```python
from build123d import *

# Parameters (mm, degrees)
SKETCH1_W           = 1500
SKETCH1_H           = 400
BOSS_EXTRUDE1_DEPTH = 6
BOSS_EXTRUDE2_DEPTH = 500
SKETCH3_W           = 10
SKETCH3_H           = 500
CUT_EXTRUDE1_DEPTH  = 4


with BuildPart() as part:
    # Sketch1 → Boss-Extrude1 (new, symmetric)
    with BuildSketch(Plane(origin=(0, 0, 0), x_dir=(1, 0, 0), z_dir=(0, 1, 0))):
        Rectangle(SKETCH1_W, SKETCH1_H)
    extrude(amount=BOSS_EXTRUDE1_DEPTH, both=True)

    # Sketch2 → Boss-Extrude2 (add)
    with BuildSketch(Plane(origin=(0, 6, 0), x_dir=(1, 0, 0), z_dir=(0, 1, 0))):
        Polygon((738, 188), (750, 188), (750, 200), (-750, 200), (-750, -200), (750, -200), (750, -188), (738, -188), (-738, -188), (-738, 188), align=None)
    extrude(amount=BOSS_EXTRUDE2_DEPTH)

    # Sketch3 → Cut-Extrude1 (cut)
    with BuildSketch(Plane.XY.offset(-188)):
        with Locations((440.2, 256)):
            Rectangle(SKETCH3_W, SKETCH3_H)
    cut_extrude1 = extrude(amount=-CUT_EXTRUDE1_DEPTH, mode=Mode.SUBTRACT)

    # Mirror1: Cut-Extrude1 across plane
    add(cut_extrude1.mirror(Plane.XY), mode=Mode.SUBTRACT)


solid = part.part
```
Part model, mm, in its own coordinate system. A direction names the side the tool comes from. Coordinates: 2 decimals unless noted, no trailing zeros. Write each loop counter-clockwise with the first axis right and the second up, starting at its lowest first coordinate (ties: lowest second). Pieces come first, ordered by that corner, then holes.
Item 1: Slice it at B-B (z = -5). Write the cut outline in (x, y), and give its area (3 significant figures).
Item 2: Mould opens along Z. For faces 1 (the face through (-143, 252, 188)), 2 (the face through (-10, 254, 200)), 3 (the face through (-4, 506, -194)), 4 (the face through (10, 246, -200)) say: released by +Z, released by -Z, zero draft, split by the parting line, or undercut.
Item 3: Which spindle directions (+Z, -Z, +X, -X, +Y, -Y) get a long thin tool onto all of the face, cutting with end or side? Do faces 5 (the face through (-10, -6, -3)), 6 (the face through (-738, 252, 3)). Say none if no direction does.
Item 4: Slice it at A-A (x = 526). Write the cut outline in (y, z), and give its area (3 significant figures).
Item 5: Probe line 1 (Z direction, x = -198, y = 236.5); line 2 (Y direction, x = 498.5, z = -60); line 3 (X direction, y = 97, z = -142). List the from-to ranges inside material, lowest first.
Item 6: Pin check, flat tips, straight feed: pin 1 (5 mm diameter, centred on x = -85, z = -72.5, fed in from +Y); pin 2 (10 mm diameter, centred on y = 222.5, z = 146.5, fed in from +X). Stop position of each tip, or through.
Item 7: Slice it at C-C (y = 182). Write the cut outline in (x, z), and give its area (3 significant figures).
Results found:
1. outline: (-750, -6) - (750, -6) - (750, 6) - (-738, 6) - (-738, 506) - (-750, 506) - close
1. area: 24,000 mm2
2. face 1: undercut
2. face 2: released by +Z
2. face 3: zero draft
2. face 4: released by -Z
3. face 5: +Z, -Z, +X, -X, -Y
3. face 6: +X, +Y
4. outline: (-6, -200) - (506, -200) - (506, -188) - (6, -188) - (6, 188) - (506, 188) - (506, 200) - (-6, 200) - close
4. area: 16,800 mm2
5. line 1: z = -200 to -188, 188 to 200
5. line 2: y = -6 to 6
5. line 3: x = -750 to -738
6. pin 1: stops at y = 6
6. pin 2: stops at x = -738
7. outline: (-750, -200) - (750, -200) - (750, -188) - (445.2, -188) - (445.2, -192) - (435.2, -192) - (435.2, -188) - (-738, -188) - (-738, 188) - (435.2, 188) - (435.2, 192) - (445.2, 192) - (445.2, 188) - (750, 188) - (750, 200) - (-750, 200) - close
7. area: 40,400 mm2
